The model under review builds one solid part; all positions refer to its coordinate system, in mm. Face numbers are marked on the shaded views. A direction names the side the tool comes from. Give positions to 0.01 mm unless a question says otherwise; leave off trailing zeros. Order: outer loops, then holes, each group sorted by start corner. A loop starts at its lowest first (then second) coordinate and runs counter-clockwise, first axis right, second up. Notation, with made-up numbers: M -16,85 L 1,85 A8 cw 1,94 Z; hole C -5,-19 d10. An arc over 180 degrees is marked long. One line per question, with ' | ' between items. Start each with the question number.
1. Wall thickness on L1, parallel to X at y = 5, z = 6.5; L2, parallel to X at y = 1.5, z = 30.5; L3, parallel to Z at x = 8.5, y = 8: over which ranges is each line inside the solid? List them lowest first.
2. We need section D-D on x = 6.5. Write out the cut boundary in (y, z), then the cut area to 3 significant figures.
3. Insertion check: P1, Ø1.9, axis at x = 5.5, z = -6.5, coming from the +Y side; P2, Ø7.5, axis at x = -2.5, y = 5, coming from the +Z side; P3, Ø0.8, axis at y = 9.5, z = -8, coming from the -X side; P4, Ø1, axis at x = 12, z = -4, coming from the -Y side. Each pin has a flat end and moves straight along its axis. Give the tip position at first contact, or say it passes through.
4. We need section A-A on z = 35. Write out the cut boundary in (x, y).
5. We need section C-C on y = 4. Write out the cut boundary in (x, z).
6. For the marked faces 1, 2, 3 and 4, list the 3-axis set-ups (+Z, -Z, +X, -X, +Y, -Y) from which the entire face can be reached by the end or side of a thin tool; tool diameter is ignored.
7. We need section B-B on z = -4. Write out the cut boundary in (x, y).
8. The part is to be moulded in two halves that separate along Y. For the marked faces 5, 6 and 7, say which applies: +Y half, -Y half, draft (parallel to the pull), parting line (faces both ways), or undercut.
```python
from build123d import *

# Parameters (mm, degrees)
F0_W      = 28.5
F0_H      = 28.5
F1_DEPTH  = 25
F3_START  = -3.2
F3_DEPTH  = 22.1
F4_DEPTH  = 18.4
F5_R      = 5
F6_R      = 3.3
F7_DEPTH  = 32.401
F8_R      = 2
F9_W      = 1
F9_H      = 6.4
F9_W_2    = 6.4
F9_H_2    = 1
F10_DEPTH = 11.8
F11_SIZE  = 1


with BuildPart() as f1:
    # F0 (on Top) → F1 (new body)
    with BuildSketch(Plane.XY):
        Rectangle(F0_W, F0_H)
    extrude(amount=F1_DEPTH)

    # F2 (on face) → F3 (join)
    with BuildSketch(Plane.XZ.offset(14.25).offset(F3_START)):
        Polygon((18.15, 23), (14.25, 23), (14.25, 7.7921073123), align=None)
    extrude(amount=-F3_DEPTH)

    # F4 (add): a face of the model
    f4_faces = [f1.faces().sort_by_distance(p)[0] for p in [
        (16.2, 0, 23),
    ]]
    extrude(f4_faces, amount=F4_DEPTH)

    # F5
    f5_edges = [f1.edges().sort_by_distance(p)[0] for p in [
        (16.2, -11.05, 41.4),
        (16.2, 11.05, 41.4),
    ]]
    fillet(f5_edges, radius=F5_R)

    # F6 (on face) → F7 (cut, through all)
    with BuildSketch(Plane.YZ.offset(18.15)):
        with Locations((0, 35)):
            Circle(F6_R)
    extrude(amount=-F7_DEPTH, mode=Mode.SUBTRACT)

    # F8
    f8_edges = [f1.edges().sort_by_distance(p)[0] for p in [
        (0, 14.25, 25),
        (-14.25, 0, 25),
        (0, -14.25, 25),
        (-14.25, 14.25, 12.5),
        (-14.25, -14.25, 12.5),
        (14.25, 14.25, 12.5),
        (14.25, -14.25, 12.5),
    ]]
    fillet(f8_edges, radius=F8_R)

    # F9 (on face) → F10 (join)
    with BuildSketch(Plane(origin=(0, 0, 0), x_dir=(1, 0, 0), z_dir=(0, 0, -1))):
        with Locations((-10.2151967585, 0)):
            Rectangle(F9_W, F9_H)
        with Locations((6.8018482998, 0)):
            Rectangle(F9_W_2, F9_H_2)
        with Locations((0, -9.5080761239)):
            Rectangle(F9_W_2, F9_H_2)
        with Locations((0, 9.7670005634)):
            Rectangle(F9_W_2, F9_H_2)
    extrude(amount=F10_DEPTH)

    # F11
    f11_edges = [f1.edges().sort_by_distance(p)[0] for p in [
        (-3.2, 9.508076, -11.8),
        (3.2, 9.508076, -11.8),
        (-10.215197, 3.2, -11.8),
        (-10.215197, -3.2, -11.8),
        (-3.2, -9.767001, -11.8),
        (3.2, -9.767001, -11.8),
        (3.601848, 0, -11.8),
        (10.001848, 0, -11.8),
    ]]
    chamfer(f11_edges, length=F11_SIZE)


solid = f1.part
```
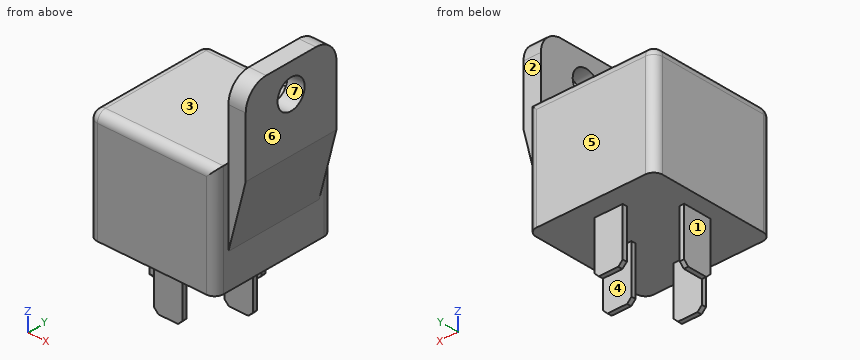
Entries:
1) L1: x = -14.25 to 14.25 | L2: x = 14.25 to 18.15 | L3: z = 0 to 25
2) outline: M -14.25,0 L -0.5,0 L -0.5,-11.8 L 0.5,-11.8 L 0.5,0 L 14.25,0 L 14.25,23 A2 ccw 12.25,25 L -12.25,25 A2 ccw -14.25,23 Z | area: 723 mm^2
3) P1: stops at y = 0.5 | P2: stops at z = 25 | P3: stops at x = -3.2 | P4: passes through
4) outline: M 14.25,-11.05 L 18.15,-11.05 L 18.15,-3.3 L 14.25,-3.3 Z; M 14.25,3.3 L 18.15,3.3 L 18.15,11.05 L 14.25,11.05 Z
5) outline: M -14.25,0 L 14.25,0 L 14.25,7.79 L 18.15,23 L 18.15,41.4 L 14.25,41.4 L 14.25,25 L -12.25,25 A2 ccw -14.25,23 Z
6) face 1: -Z, -X, +Y, -Y | face 2: +Z, -Z, +X, +Y | face 3: +Z, -X, +Y, -Y | face 4: -Z, +X, +Y
7) outline: M -10.72,-3.2 L -9.72,-3.2 L -9.72,3.2 L -10.72,3.2 Z; M -3.2,-10.27 L 3.2,-10.27 L 3.2,-9.27 L -3.2,-9.27 Z; M -3.2,9.01 L 3.2,9.01 L 3.2,10.01 L -3.2,10.01 Z; M 3.6,-0.5 L 10,-0.5 L 10,0.5 L 3.6,0.5 Z
8) face 5: +Y half | face 6: draft | face 7: undercut
